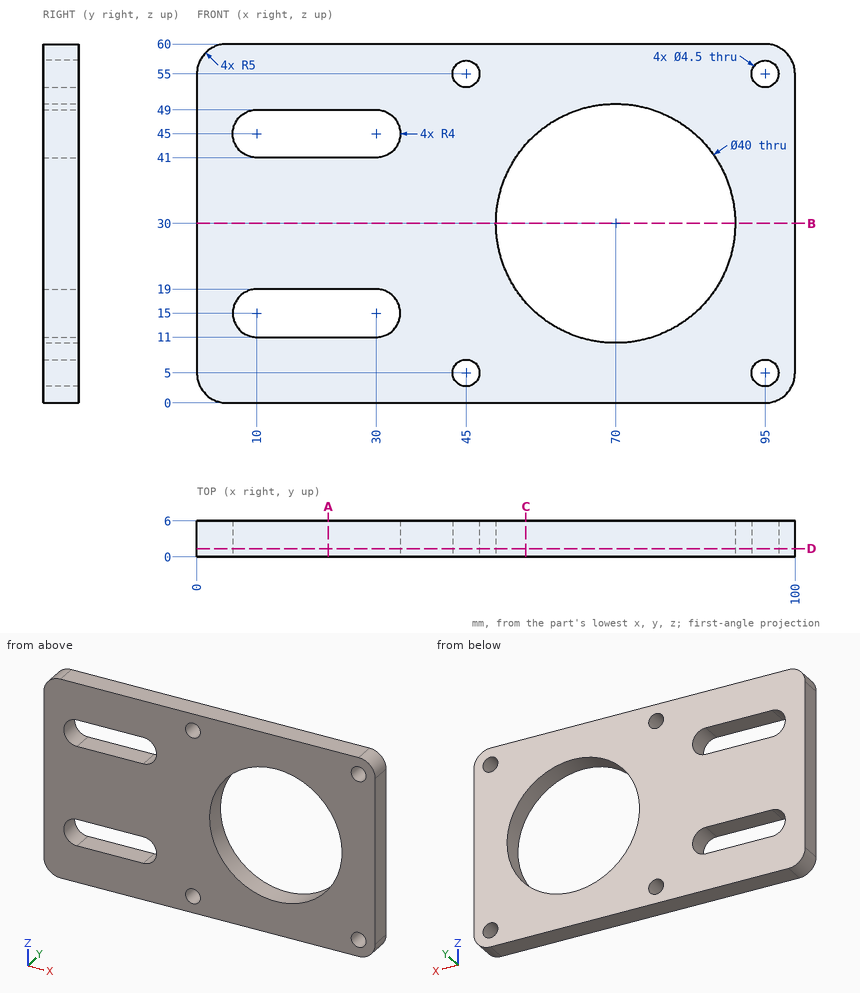
For this review, use the dimensioned drawing (mm, ordinates from the lowest corner) and the shaded views. Round coordinates to 2 decimals unless told otherwise and drop trailing zeros. Order: outer loops, then holes, each group sorted by start corner. A loop starts at its lowest first (then second) coordinate and runs counter-clockwise, first axis right, second up.
1) Clearance check with a flat-ended pin moving along its axis: pin 1 Ø5 at (x, z) = (45, 55) entering from +Y. State where the tip first meets the part, or that it passes through.
The answers:
pin 1: stops at y = 6
2) Consider section D-D (y = 1.35). State the section outline as (x, z) points, plus the area to 3 significant figures.
The answers:
outline: (0, 5) arc R5 ccw to (5, 0) - (95, 0) arc R5 ccw to (100, 5) - (100, 55) arc R5 ccw to (95, 60) - (5, 60) arc R5 ccw to (0, 55) - close; hole (10, 11) - (30, 11) arc R4 ccw to (30, 19) - (10, 19) arc R4 ccw to start; hole (10, 41) - (30, 41) arc R4 ccw to (30, 49) - (10, 49) arc R4 ccw to start; hole circle Ø4.5 at (45, 5); hole circle Ø4.5 at (45, 55); hole circle Ø40 at (70, 30); hole circle Ø4.5 at (95, 5); hole circle Ø4.5 at (95, 55)
area: 4,240 mm2
3) For L1, parallel to Z at x = 25.5, y = 1.65; L2, parallel to X at y = 2.5, z = 30; L3, parallel to X at y = 5.7, z = 15.5, list the stretches that pass through material, from the lowest coordinate up.
The answers:
L1: z = 0 to 11, 19 to 41, 49 to 60
L2: x = 0 to 50, 90 to 100
L3: x = 0 to 6.03, 33.97 to 56.23, 83.77 to 100
4) Consider section C-C (x = 55). State the section outline as (y, z) points, plus the area to 3 significant figures.
The answers:
outline: (0, 0) - (6, 0) - (6, 16.77) - (0, 16.77) - close; (0, 43.23) - (6, 43.23) - (6, 60) - (0, 60) - close
area: 201 mm2
5) Consider section A-A (x = 22). State the section outline as (y, z) points.
The answers:
outline: (0, 0) - (6, 0) - (6, 11) - (0, 11) - close; (0, 19) - (6, 19) - (6, 41) - (0, 41) - close; (0, 49) - (6, 49) - (6, 60) - (0, 60) - close
6) Consider section B-B (z = 30). State the section outline as (x, y) points, plus the area to 3 significant figures.
The answers:
outline: (0, 0) - (50, 0) - (50, 6) - (0, 6) - close; (90, 0) - (100, 0) - (100, 6) - (90, 6) - close
area: 360 mm2
